The listing builds one solid part. Answer for the finished solid, in the listing's coordinates (mm). A direction names the side the tool comes from. Round coordinates to 2 decimals unless told otherwise and drop trailing zeros. Loops run counter-clockwise (first coordinate to the right, second up) from the corner with the lowest first, then second, coordinate; pieces in that order, holes last. Notation, with made-up numbers: (78, 72.5) -> (135, 72.5) arc R20 cw to (135, 88.5) -> close; hole circle Ø7 at (7.25, -11.5). An arc over 180 degrees is marked (long way). Answer in a Markdown table with one row per item. Add a question column.
```python
from build123d import *

# Parameters (mm, degrees)
F0_W     = 25.4
F0_H     = 25.4
F1_DEPTH = 5


with BuildPart() as f1:
    # F0 (on Front) → F1 (new body)
    with BuildSketch(Plane.XZ):
        with Locations((46.112889, 54.660929)):
            Rectangle(F0_W, F0_H)
        with BuildLine():
            ThreePointArc((55.573677, 63.996648), (56.045747, 63.095671), (56.208677, 62.091648))
            ThreePointArc((56.208677, 62.091648), (52.029654, 59.079578), (50.493677, 63.996648))
            ThreePointArc((50.493677, 63.996648), (53.033677, 65.266648), (55.573677, 63.996648))
        make_face(mode=Mode.SUBTRACT)
        with BuildLine():
            Line((50.493677, 63.996648), (55.573677, 63.996648))
            ThreePointArc((55.573677, 63.996648), (53.033677, 65.266648), (50.493677, 63.996648))
        make_face()
    extrude(amount=F1_DEPTH)


solid = f1.part
```
Item 1: Consider L1, parallel to Z at x = 53, y = -1.1; L2, parallel to X at y = -0.5, z = 62; L3, parallel to Z at x = 51, y = -2.75. Determine where each line is inside the solid, lowest interval first. Write a range as from..to.
Item 2: For faces 1 (the flat face through (53, -2, 63.997)), 2 (the flat face through (46, 0, 55)), determine the directions among +Z, -Z, +X, -X, +Y, -Y from which every point of the face is accessible in a straight line to the end or side of a thin tool.
Item 3: Section A-A, the plane y = -3.3 is taken. Write down the section's boundary in (x, z) (3 decimals).
Here are the results:
| question | item | result |
|---|---|---|
| 1 | L1 | z = 41.96..58.92, 64..67.36 |
| 1 | L2 | x = 33.41..49.86, 56.21..58.81 |
| 1 | L3 | z = 41.96..59.65, 64..67.36 |
| 2 | face 1 | +Y, -Y |
| 2 | face 2 | +Z, -Z, +X, -X, +Y |
| 3 | outline | (33.413, 41.961) -> (58.813, 41.961) -> (58.813, 67.361) -> (33.413, 67.361) -> close; hole (50.494, 63.997) arc R3.175 ccw (long way) to (56.209, 62.092) arc R3.175 ccw to (55.574, 63.997) -> close |
